For this review, take the finished solid that the model builds, in its own axes (mm). A direction names the side the tool comes from. Give positions to 0.01 mm unless a question says otherwise; leave off trailing zeros. Order: outer loops, then holes, each group sorted by start corner. A loop starts at its lowest first (then second) coordinate and runs counter-clockwise, first axis right, second up. Notation, with made-up numbers: M 43,4.25 L 54,4.25 A19 ccw 54,30.25 Z; hole C 36.5,0 d1. An arc over 180 degrees is marked long. Use CSV: the item, a comma, the result in double quotes. Start each with the question number.
(1) Tool access review of faces 5 (the face through (-1, -13.5, 0)), 6 (the face through (-1, 16, 2.75)), 7 (the face through (9, 0, -3)): name each direction out of +Z, -Z, +X, -X, +Y, -Y from which nothing blocks a thin tool from reaching the whole face with its end or side.
(2) Consider section D-D (y = 15.5). Write out the cut boundary in (x, z).
(3) Consider section B-B (x = -3). Write out the cut boundary in (y, z).
(4) Draft analysis for pull direction X (two halves, no side actions). For faces 1 (the face through (-87.312, -1, -3)), 2 (the face through (-1, 12.5, 0)), 3 (the face through (87.312, -1, -3)), 4 (the face through (41, 0, -3)), state which applies: pulls with the +X half, pulls with the -X half, needs draft (parallel to the pull), parting line crosses it, or undercut.
(5) Clearance check with flat-ended pins moving along their axes: P1, Ø0.8, axis at x = 22, z = -3, coming from the -Y side; P2, Ø0.5, axis at x = 52, z = -3, coming from the +Y side; P3, Ø0.5, axis at x = 74, z = -3.5, coming from the -Y side. State where each tip first meets the part, or that it passes through.
(6) Wall thickness on L1, parallel to Y at x = 36, z = 1.5; L2, parallel to Z at x = 15.5, y = 3; L3, parallel to Z at x = 46, y = -15: over which ranges is each line inside the solid? List them lowest first. Write a range as from..to.
(7) Consider section A-A (z = -0.5). Write out the cut boundary in (x, y).
(8) Consider section C-C (y = 0). Give the number of separate pieces and of enclosed holes in the cut face, and give its area (3 significant figures).
```python
from build123d import *

# Parameters (mm, degrees)
EXTRUDE_THIN1_DEPTH      = 87.3125
EXTRUDE_THIN1_DEPTH_BACK = 87.3125
CUT_EXTRUDE1_DEPTH       = 90.127914574
LPATTERN1_COUNT          = 4
LPATTERN1_PITCH          = 25
LPATTERN1_COL_COUNT      = 4
LPATTERN1_COL_PITCH      = 25


with BuildPart() as part:
    # Sketch3 → Extrude-Thin1 (new, two sides: drawn at the far end of the back side and taken through both)
    with BuildSketch(Plane(origin=(0, 0, 0), x_dir=(0, 0, -1), z_dir=(1, 0, 0)).offset(-EXTRUDE_THIN1_DEPTH_BACK)):
        with BuildLine():
            Line((-2.75, -17.5), (-2.75, -14))
            ThreePointArc((-2.75, -14), (-2.603553391, -13.646446609), (-2.25, -13.5))
            Line((-2.25, -13.5), (2.25, -13.5))
            ThreePointArc((2.25, -13.5), (3.310660172, -13.060660172), (3.75, -12))
            Line((3.75, -12), (3.75, 12))
            ThreePointArc((3.75, 12), (3.310660172, 13.060660172), (2.25, 13.5))
            Line((2.25, 13.5), (-2.25, 13.5))
            ThreePointArc((-2.25, 13.5), (-2.603553391, 13.646446609), (-2.75, 14))
            Line((-2.75, 14), (-2.75, 17.5))
            Line((-2.75, 17.5), (-3.75, 17.5))
            Line((-3.75, 17.5), (-3.75, 14))
            ThreePointArc((-3.75, 14), (-3.310660172, 12.939339828), (-2.25, 12.5))
            Line((-2.25, 12.5), (2.25, 12.5))
            ThreePointArc((2.25, 12.5), (2.603553391, 12.353553391), (2.75, 12))
            Line((2.75, 12), (2.75, -12))
            ThreePointArc((2.75, -12), (2.603553391, -12.353553391), (2.25, -12.5))
            Line((2.25, -12.5), (-2.25, -12.5))
            ThreePointArc((-2.25, -12.5), (-3.310660172, -12.939339828), (-3.75, -14))
            Line((-3.75, -14), (-3.75, -17.5))
            Line((-3.75, -17.5), (-2.75, -17.5))
        make_face()
    extrude(amount=EXTRUDE_THIN1_DEPTH + EXTRUDE_THIN1_DEPTH_BACK)

    # Sketch4 → Cut-Extrude1 (cut, through all)
    with BuildSketch(Plane.XY):
        with BuildLine():
            Line((-5.85, -3.15), (5.85, -3.15))
            ThreePointArc((5.85, -3.15), (9, 0), (5.85, 3.15))
            Line((5.85, 3.15), (-5.85, 3.15))
            ThreePointArc((-5.85, 3.15), (-9, 0), (-5.85, -3.15))
        make_face()
    cut_extrude1 = extrude(amount=-CUT_EXTRUDE1_DEPTH, mode=Mode.SUBTRACT)

    # LPattern1: Cut-Extrude1 ×4
    with Locations(*[(i * LPATTERN1_PITCH, 0, 0) for i in range(1, LPATTERN1_COUNT)]):
        add(cut_extrude1, mode=Mode.SUBTRACT)

    # LPattern1 col: Cut-Extrude1 ×4
    with Locations(*[(-i * LPATTERN1_COL_PITCH, 0, 0) for i in range(1, LPATTERN1_COL_COUNT)]):
        add(cut_extrude1, mode=Mode.SUBTRACT)


solid = part.part
```
Check result:
1,face 5,"-Z, +X, -X, -Y"
1,face 6,"-Z, +X, -X, +Y"
1,face 7,"+Z, -Z"
2,outline,"M -87.31,2.75 L 87.31,2.75 L 87.31,3.75 L -87.31,3.75 Z"
3,outline,"M -17.5,2.75 L -14,2.75 A0.5 cw -13.5,2.25 L -13.5,-2.25 A1.5 ccw -12,-3.75 L -3.15,-3.75 L -3.15,-2.75 L -12,-2.75 A0.5 cw -12.5,-2.25 L -12.5,2.25 A1.5 ccw -14,3.75 L -17.5,3.75 Z; M 3.15,-3.75 L 12,-3.75 A1.5 ccw 13.5,-2.25 L 13.5,2.25 A0.5 cw 14,2.75 L 17.5,2.75 L 17.5,3.75 L 14,3.75 A1.5 ccw 12.5,2.25 L 12.5,-2.25 A0.5 cw 12,-2.75 L 3.15,-2.75 Z"
4,face 1,"pulls with the -X half"
4,face 2,"needs draft"
4,face 3,"pulls with the +X half"
4,face 4,"undercut"
5,P1,"stops at y = -13.46"
5,P2,"stops at y = 13.41"
5,P3,"stops at y = -13.12"
6,L1,"y = -13.5..-12.5, 12.5..13.5"
6,L2,"z = -3.75..-2.75"
6,L3,"z = 2.75..3.75"
7,outline,"M -87.31,-13.5 L 87.31,-13.5 L 87.31,-12.5 L -87.31,-12.5 Z; M -87.31,12.5 L 87.31,12.5 L 87.31,13.5 L -87.31,13.5 Z"
8,separate pieces,"8"
8,enclosed holes,"0"
8,area,"48.6 mm^2"
